Geometry check sheet. Reference: drawing and pictorial views, mm from the part's lowest x, y, z. A direction names the side the tool comes from. Give positions to 0.01 mm unless a question says otherwise; leave off trailing zeros. Order: outer loops, then holes, each group sorted by start corner. A loop starts at its lowest first (then second) coordinate and runs counter-clockwise, first axis right, second up. Notation, with made-up numbers: (61, -8) - (95, -8) arc R32 ccw to (95, 22) - close; hole circle Ø9 at (62.25, -1). An arc over 180 degrees is marked (long way). Answer as a JSON object with one key per item and string values.
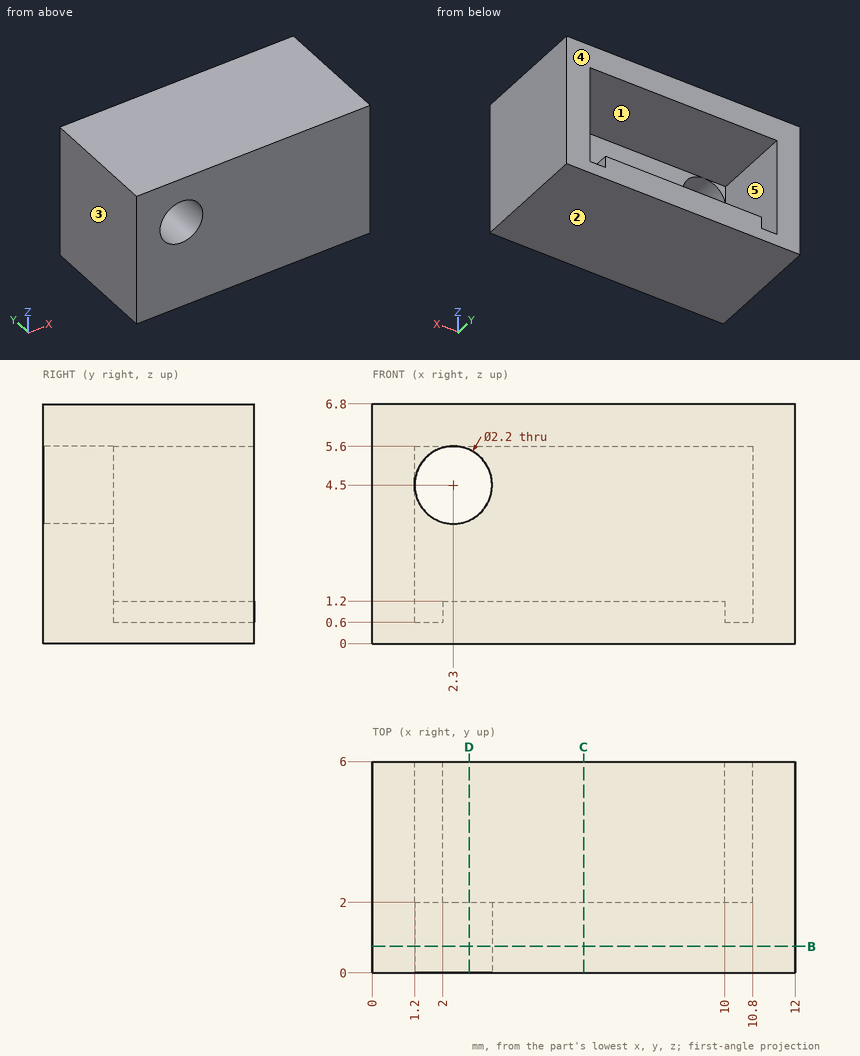
(1) Release check for a two-part mould opening along X. For the marked faces 1, 2 and 3 record: pulls with the +X half, pulls with the -X half, needs draft (parallel to the pull), parting line crosses it, or undercut.
Computed values:
{"face 1": "undercut", "face 2": "needs draft", "face 3": "pulls with the -X half"}
(2) Section check D-D (x = 2.75). Record the cut outline in (y, z).
Computed values:
{"outline": "(0, 0) - (6, 0) - (6, 1.2) - (2, 1.2) - (2, 3.5) - (0, 3.5) - close; (0, 5.5) - (2, 5.5) - (2, 5.6) - (6, 5.6) - (6, 6.8) - (0, 6.8) - close"}
(3) Access from +Z, -Z, +X, -X, +Y, -Y to the whole of each face (thin tool, end or side, straight path). Record for the marked faces 4 and 5.
Computed values:
{"face 4": "+Z, -Z, +X, -X, +Y", "face 5": "+Y"}
(4) Section check B-B (y = 0.75). Record the cut outline in (x, z), then the cut area to 3 significant figures.
Computed values:
{"outline": "(0, 0) - (12, 0) - (12, 6.8) - (0, 6.8) - close; hole circle Ø2.2 at (2.3, 4.5)", "area": "77.8 mm²"}
(5) Gauge pin test, flat end, axial feed: pin 1 Ø1.5 at (x, z) = (5, 2) entering from +Y. Record the tip position at first contact, or that the pin passes through.
Computed values:
{"pin 1": "stops at y = 2"}
(6) Material ranges on line 1 along X through (y, z) = (5.25, 1.75); line 2 along X through (y, z) = (1.15, 4.5); line 3 along Z through (x, y) = (2.3, 0.85), recorded low to high. Write a range as [from, to].
Computed values:
{"line 1": "x = [0, 1.2], [10.8, 12]", "line 2": "x = [0, 1.2], [3.4, 12]", "line 3": "z = [0, 3.4], [5.6, 6.8]"}
(7) Section check C-C (x = 6). Record the cut outline in (y, z), then the cut area to 3 significant figures.
Computed values:
{"outline": "(0, 0) - (6, 0) - (6, 1.2) - (2, 1.2) - (2, 5.6) - (6, 5.6) - (6, 6.8) - (0, 6.8) - close", "area": "23.2 mm²"}
